Check sheet for the drawn part. Datum: minimum x, y, z corner. Units: mm. A direction names the side the tool comes from. Give positions to 0.01 mm unless a question says otherwise; leave off trailing zeros. Write each loop counter-clockwise with the first axis right and the second up, starting at its lowest first coordinate (ties: lowest second). Pieces come first, ordered by that corner, then holes.
(1) Depth check by flat-ended pin: P1, Ø3, axis at x = 1.5, y = 5, coming from the +Z side; P2, Ø4, axis at x = 3.5, y = 19.5, coming from the +Z side. Enter the tip coordinate at first touch or a pass-through.
(2) Cross-section at B-B (y = 22.5). Record the boundary of the cut face in (x, z).
(3) Thickness scan on line 1 along Z through (x, y) = (2.75, 3.5); line 2 along Z through (x, y) = (3.75, 5.5); line 3 along Y through (x, z) = (7.5, 31.5). Record the ranges inside material, lowest first.
(4) Cross-section at C-C (z = 29.5). Record the boundary of the cut face in (x, y).
(5) Tool access check on the marked faces 1 and 2. Record the directions out of +Z, -Z, +X, -X, +Y, -Y that give a thin tool (end or side, any length) a straight path to the whole face; none if there is none.
(6) Cross-section at A-A (x = 6.25). Record the boundary of the cut face in (y, z).
(7) Cross-section at D-D (x = 10.5). Record the boundary of the cut face in (y, z) (1 decimal).
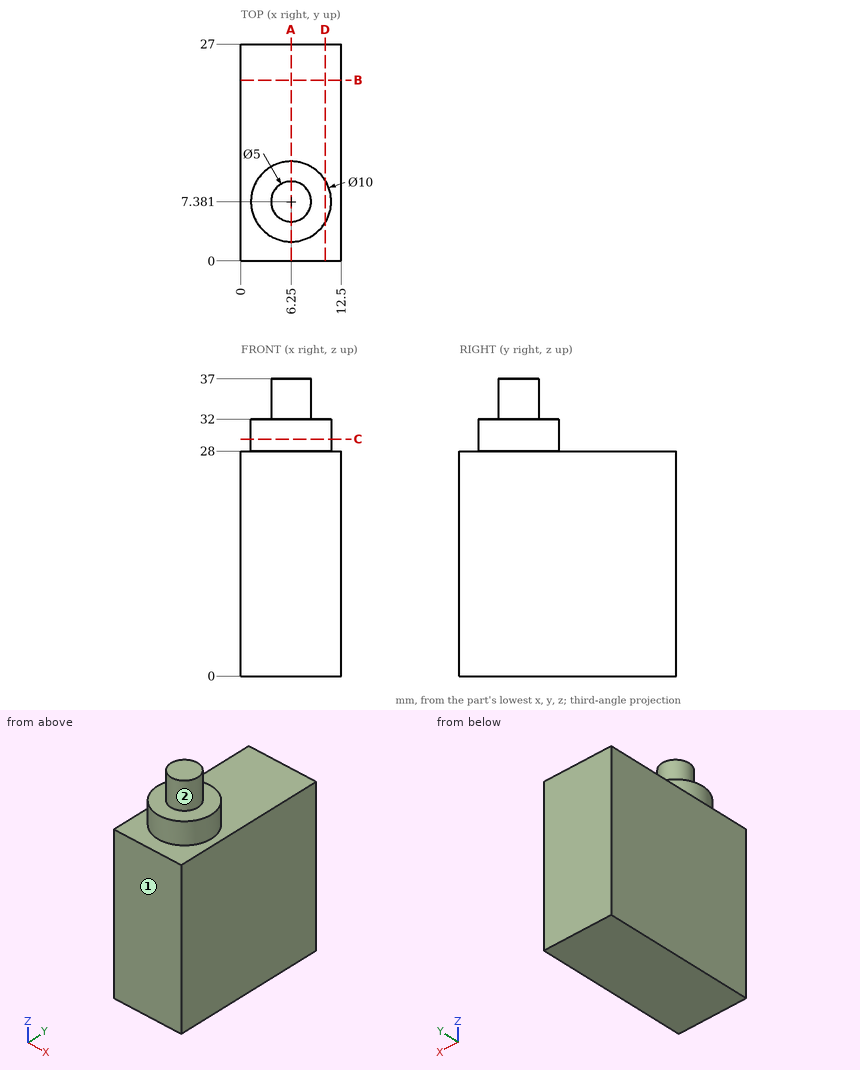
Reply:
1. P1: stops at z = 32
1. P2: stops at z = 28
2. outline: (0, 0) - (12.5, 0) - (12.5, 28) - (0, 28) - close
3. line 1: z = 0 to 28
3. line 2: z = 0 to 32
3. line 3: y = 2.54 to 12.22
4. outline: circle Ø10 at (6.25, 7.38)
5. face 1: +Z, -Z, +X, -X, -Y
5. face 2: +Z
6. outline: (0, 0) - (27, 0) - (27, 28) - (12.38, 28) - (12.38, 32) - (9.88, 32) - (9.88, 37) - (4.88, 37) - (4.88, 32) - (2.38, 32) - (2.38, 28) - (0, 28) - close
7. outline: (0, 0) - (27, 0) - (27, 28) - (10, 28) - (10, 32) - (4.7, 32) - (4.7, 28) - (0, 28) - close
